Here's how the part is built. I have some questions about the finished solid (model axes, mm). A direction names the side the tool comes from. Coordinates: 2 decimals unless noted, no trailing zeros. Write each loop counter-clockwise with the first axis right and the second up, starting at its lowest first coordinate (ties: lowest second). Pieces come first, ordered by that corner, then holes. Notation, with made-up numbers: (20, 15.5) -> (30, 15.5) arc R16 cw to (30, 35.5) -> close; hole circle Ø8 at (25.5, 82.5). An arc over 180 degrees is marked (long way). Put each result on its own line as item: value. Start each with the question number.
Item 1: I need wall thicknesses on line 1 (Y direction, x = 0, z = -14); line 2 (Z direction, x = 0, y = -62.5); line 3 (X direction, y = -41, z = 6). Which ranges of each line are inside material? Lowest first, please. Write a range as [from, to].
Item 2: I want a section at C-C, the plane z = -30.5. List the corners of the cut face in (x, y) for me, then the cut area to 3 significant figures.
Item 3: If we mould it in two halves opening along X, with no side actions, what happens to faces 3 (the face through (-8, -55, -24)), 4 (the face through (-1.107, -47.821, 8.428)), 5 (the face through (0, -40.8, -40))? For each: released by +X, released by -X, zero draft, split by the parting line, or undercut.
Item 4: I want a section at A-A, the plane x = 0. List the corners of the cut face in (y, z) for me.
Item 5: For pin 1 (8 mm diameter, centred on x = -5, y = -61, fed in from +Z); pin 2 (3 mm diameter, centred on x = -2.5, z = -24.5, fed in from +Y); pin 3 (2 mm diameter, centred on x = -4, y = -11, fed in from +Z), each with a flat end and sliding along its axis, tell me the tip position at first contact or that it passes through.
Item 6: On a 3-axis mill with a long thin cutter (end or side, diameter ignored), from which of +Z, -Z, +X, -X, +Y, -Y can I reach the whole of each face in a straight line? I mean faces 1 (the face through (-1.302, -47.821, 9.915)), 2 (the face through (-4.5, 0, -7.4)). Say none if no direction works.
Item 7: I want a section at D-D, the plane z = 4. List the corners of the cut face in (x, y) for me, then the cut area to 3 significant figures.
Item 8: I want a section at B-B, the plane y = -49. List the corners of the cut face in (x, z) for me.
from build123d import *

# Parameters (mm, degrees)
F0_R     = 10
F0_R_2   = 8.5
F1_DEPTH = 97
F2_R     = 10
F2_R_2   = 8
F3_DEPTH = 40
F4_R     = 8
F5_DEPTH = 59.3
F6_R     = 8.5
F7_DEPTH = 110


with BuildPart() as f1:
    # F0 (on Front) → F1 (new body)
    with BuildSketch(Plane.XZ):
        Circle(F0_R)
        Circle(F0_R_2, mode=Mode.SUBTRACT)
    extrude(amount=F1_DEPTH)

    # F2 (on Top) → F3 (join)
    with BuildSketch(Plane.XY):
        with Locations((0, -49)):
            Circle(F2_R)
        with Locations((0, -49)):
            Circle(F2_R_2, mode=Mode.SUBTRACT)
    extrude(amount=-F3_DEPTH)

    # F4 (on Top) → F5 (cut)
    with BuildSketch(Plane.XY):
        with Locations((0, -49)):
            Circle(F4_R)
    extrude(amount=-F5_DEPTH, mode=Mode.SUBTRACT)

    # F6 (on Front) → F7 (cut)
    with BuildSketch(Plane.XZ):
        Circle(F6_R)
    extrude(amount=F7_DEPTH, mode=Mode.SUBTRACT)


solid = f1.part
Calculated:
1. line 1: y = [-59, -57], [-41, -39]
1. line 2: z = [-10, -8.5], [8.5, 10]
1. line 3: x = [-8, -6.02], [6.02, 8]
2. outline: circle Ø20 at (0, -49); hole circle Ø16 at (0, -49)
2. area: 113 mm2
3. face 3: split by the parting line
3. face 4: undercut
3. face 5: zero draft
4. outline: (-97, -10) -> (-59, -10) -> (-59, -40) -> (-57, -40) -> (-57, -8.5) -> (-97, -8.5) -> close; (-97, 8.5) -> (0, 8.5) -> (0, 10) -> (-97, 10) -> close; (-41, -40) -> (-39, -40) -> (-39, -10) -> (0, -10) -> (0, -8.5) -> (-41, -8.5) -> close
5. pin 1: stops at z = 9.95
5. pin 2: stops at y = -39.05
5. pin 3: stops at z = 9.54
6. face 1: none
6. face 2: +Z, -Z, +X, -X, +Y
7. outline: (-9.17, -97) -> (-7.5, -97) -> (-7.5, 0) -> (-9.17, 0) -> close; (7.5, -97) -> (9.17, -97) -> (9.17, 0) -> (7.5, 0) -> close
7. area: 323 mm2
8. outline: (-10, -40) -> (-8, -40) -> (-8, -2.87) arc R8.5 cw (long way) to (8, -2.87) -> (8, -40) -> (10, -40) -> (10, 0) arc R10 ccw to (-10, 0) -> close
